from build123d import *

# Parameters (mm, degrees)
SKETCH_2_R          = 1
EXTRUDE_3_DEPTH     = 1.6
EXTRUDE_START       = 1.6
SKETCH_3_W          = 19.3
SKETCH_3_H          = 9.2
EXTRUDE_4_DEPTH     = 15.2
CUT_EXTRUDE_START   = 16.8
SKETCH_4_W          = 15.24
SKETCH_4_H          = 1.6
CUT_EXTRUDE_1_DEPTH = 9
CUT_EXTRUDE_2_DEPTH = 15.2
SKETCH_6_W          = 10.5
SKETCH_6_H          = 3.6
SKETCH_6_W_2        = 15
EXTRUDE_5_DEPTH     = 4.5


with BuildPart() as part:
    # 草图2 → 凸台-拉伸3 (new body)
    with BuildSketch(Plane(origin=(0, 0, 0), x_dir=(1, 0, 0), z_dir=(0, 1, 0))):
        with BuildLine():
            Line((-10.65, 12.5), (10.65, 12.5))
            ThreePointArc((10.65, 12.5), (11.958147545, 11.958147545), (12.5, 10.65))
            Line((12.5, 10.65), (12.5, -10.65))
            ThreePointArc((12.5, -10.65), (11.958147545, -11.958147545), (10.65, -12.5))
            Line((10.65, -12.5), (-10.65, -12.5))
            ThreePointArc((-10.65, -12.5), (-11.958147545, -11.958147545), (-12.5, -10.65))
            Line((-12.5, -10.65), (-12.5, 10.65))
            ThreePointArc((-12.5, 10.65), (-11.958147545, 11.958147545), (-10.65, 12.5))
        make_face()
        with Locations(Location((-10.65, 10.65, 0), (0, 0, 270))):
            Circle(SKETCH_2_R, mode=Mode.SUBTRACT)
        with Locations(Location((10.65, 10.65, 0), (0, 0, 270))):
            Circle(SKETCH_2_R, mode=Mode.SUBTRACT)
        with Locations(Location((-10.65, -10.65, 0), (0, 0, 270))):
            Circle(SKETCH_2_R, mode=Mode.SUBTRACT)
        with Locations(Location((10.65, -10.65, 0), (0, 0, 270))):
            Circle(SKETCH_2_R, mode=Mode.SUBTRACT)
    extrude(amount=EXTRUDE_3_DEPTH)

    # 草图3 → 凸台-拉伸4 (add)
    with BuildSketch(Plane(origin=(0, 0, 0), x_dir=(1, 0, 0), z_dir=(0, 1, 0)).offset(EXTRUDE_START)):
        Rectangle(SKETCH_3_W, SKETCH_3_H)
    extrude(amount=EXTRUDE_4_DEPTH)

    # 草图4 → 切除-拉伸1 (cut)
    with BuildSketch(Plane(origin=(0, 0, 0), x_dir=(1, 0, 0), z_dir=(0, 1, 0)).offset(CUT_EXTRUDE_START)):
        Rectangle(SKETCH_4_W, SKETCH_4_H)
    extrude(amount=-CUT_EXTRUDE_1_DEPTH, mode=Mode.SUBTRACT)

    # 草图5 → 切除-拉伸2 (cut)
    with BuildSketch(Plane(origin=(0, 0, 0), x_dir=(1, 0, 0), z_dir=(0, 1, 0)).offset(CUT_EXTRUDE_START)):
        Polygon((9.65, 4.6), (9.65, 3.6), (8.65, 4.6), align=None)
        Polygon((9.65, -4.6), (9.65, -3.6), (8.65, -4.6), align=None)
        Polygon((-9.65, -4.6), (-8.65, -4.6), (-9.65, -3.6), align=None)
        Polygon((-9.65, 4.6), (-8.65, 4.6), (-9.65, 3.6), align=None)
    extrude(amount=-CUT_EXTRUDE_2_DEPTH, mode=Mode.SUBTRACT)

    # 草图6 → 凸台-拉伸5 (add)
    with BuildSketch(Plane(origin=(0, 0, 0), x_dir=(1, 0, 0), z_dir=(0, 1, 0))):
        with Locations((0, -10.7)):
            Rectangle(SKETCH_6_W, SKETCH_6_H)
        with Locations((0, 10.7)):
            Rectangle(SKETCH_6_W_2, SKETCH_6_H)
    extrude(amount=-EXTRUDE_5_DEPTH)


solid = part.part
Geometry: final body of the model. Coordinates: model frame, mm. A direction names the side the tool comes from. Coordinates: 2 decimals unless noted, no trailing zeros. Loops run counter-clockwise (first coordinate to the right, second up) from the corner with the lowest first, then second, coordinate; pieces in that order, holes last. Notation, with made-up numbers: (-15, 24.5) - (24, 24.5) arc R35 ccw to (24, 59.5) - close; hole circle Ø10 at (11.5, -21.75). An arc over 180 degrees is marked (long way). One line per question, with ' | ' between items. Start each with the question number.
(1) Cut plane B-B on y = 8.5. Output: boundary loops of the cut face in (x, z), and give its area (3 significant figures).
(2) Cut plane C-C on x = -4. Output: boundary loops of the cut face in (y, z), and give its area (3 significant figures).
(3) Draft query along X for faces 5 (the cylindrical face through (-11.033, 0.789, -9.726)), 6 (the flat face through (-7.5, -2, -11)), 7 (the flat face through (0, 9, -4.6)), 8 (the cylindrical face through (10.69, 0.79, 9.65)). Return one class per face: +X half, -X half, draft (parallel to the pull), parting line (faces both ways), or undercut.
(4) Ray query, L1, parallel to X at y = 1.1, z = 10.65; L2, parallel to Z at x = -4.5, y = -2; L3, parallel to X at y = 13.5, z = -0.5. Return the intervals inside material, ascending. Write a range as from..to.
(5) First-contact query: pin 1 (2.5 mm diameter, centred on x = 10.65, z = 10.65, fed in from -Y); pin 2 (1.8 mm diameter, centred on x = -2.5, z = 0, fed in from +Y); pin 3 (1.8 mm diameter, centred on y = 10.5, z = 0, fed in from +X); pin 4 (0.5 mm diameter, centred on y = 11, z = 0, fed in from -X). Flat tips, straight axial feed; report the tip coordinate or a pass-through.
(6) Cut plane A-A on x = -9.25. Output: boundary loops of the cut face in (y, z), and give its area (3 significant figures).
(7) Reachability of faces 1 (the flat face through (9.16, 9.31, -4.09)), 2 (the flat face through (7.62, 12, 0)), 3 (the flat face through (0, -2, 8.9)), 4 (the flat face through (7.5, -2, -11)) from +Z, -Z, +X, -X, +Y, -Y: full face, straight path, thin tool, end or side. Return the list, or none.
Here are the results:
1) outline: (-9.65, -3.6) - (-8.65, -4.6) - (8.65, -4.6) - (9.65, -3.6) - (9.65, 3.6) - (8.65, 4.6) - (-8.65, 4.6) - (-9.65, 3.6) - close; hole (-7.62, -0.8) - (7.62, -0.8) - (7.62, 0.8) - (-7.62, 0.8) - close | area: 151 mm²
2) outline: (-4.5, -12.5) - (1.6, -12.5) - (1.6, -4.6) - (16.8, -4.6) - (16.8, -0.8) - (7.8, -0.8) - (7.8, 0.8) - (16.8, 0.8) - (16.8, 4.6) - (1.6, 4.6) - (1.6, 12.5) - (-4.5, 12.5) - (-4.5, 8.9) - (0, 8.9) - (0, -8.9) - (-4.5, -8.9) - close | area: 198 mm²
3) face 5: undercut | face 6: -X half | face 7: draft | face 8: undercut
4) L1: -12.5..-11.65, -9.65..9.65, 11.65..12.5 | L2: -12.5..-8.9, 8.9..12.5 | L3: -9.65..-7.62, 7.62..9.65
5) pin 1: y = 0 | pin 2: y = 16.8 | pin 3: x = 9.65 | pin 4: x = -9.65
6) outline: (0, -12.5) - (1.6, -12.5) - (1.6, -4) - (16.8, -4) - (16.8, 4) - (1.6, 4) - (1.6, 12.5) - (0, 12.5) - close | area: 162 mm²
7) face 1: -Z, +X, +Y | face 2: +Y | face 3: +X, -X, -Y | face 4: +Z, -Z, +X, -Y
